The listing builds one solid part. Answer for the finished solid, in the listing's coordinates (mm). Round coordinates to 2 decimals unless told otherwise and drop trailing zeros. Write each loop counter-clockwise with the first axis right and the second up, starting at its lowest first coordinate (ties: lowest second). Pieces come first, ordered by that corner, then holes.
Item 1: Find section C-C on x = 45.65. Give the vertices of the cut face in (y, z).
Item 2: Find the intervals of material crossed by probe 1 along Y at (x, z) = (76.65, 1.2); probe 2 along X at (y, z) = (36.5, 0.2); probe 3 along X at (y, z) = (36.65, 0.9), in increasing order.
Item 3: Find section A-A on x = 61.15. Give the vertices of the cut face in (y, z).
Item 4: Find section B-B on y = 26.5. Give the vertices of the cut face in (x, z), then the cut area to 3 significant figures.
Item 5: Find section D-D on z = 2.15. Give the vertices of the cut face in (x, y).
Solid Edge part; units mm, degrees
sketch "Sketch1" plane through (0, 0, 0) normal (0, 0, 1) x (1, 0, 0)
  line L0 (0, 0) -> (82.3, 0)
  line L1 (82.3, 0) -> (82.3, 42.3)
  line L2 (82.3, 42.3) -> (40, 42.3)
  line L3 (40, 42.3) -> (0, 20)
  line L4 (0, 20) -> (0, 0)
extrude "Protrusion1" add sketch "Sketch1" along normal blind 4
hole "Hole_1" at (10, 10, 4) direction (0, 0, -1) diameter 8 end up to next
hole "Hole1" at (30, 10, 4) direction (0, 0, -1) diameter 8 end up to next
hole "Hole_3" at (61.15, 21.15, 4) direction (0, 0, -1) diameter 23 end up to next
hole "Hole_4" at (45.65, 36.65, 4) direction (0, 0, -1) diameter 3.2 end up to next
pattern_linear "Pattern2" count 2 spacing 31 along (1, 0, 0) count 2 spacing 31 along (0, -1, 0) of "Hole_4"
fillet "Round_1" radius 5 4 edges at (0, 20, 2) (82.3, 42.3, 2) (82.3, 0, 2) (40, 42.3, 2)
fillet "Round_2" radius 1.5 1 edges at (0, 0, 2)
properties material "Aluminum, 6061-T6"
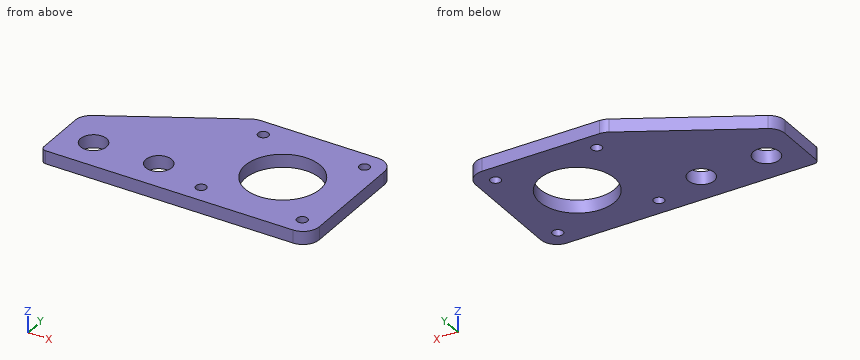
Check values:
1. outline: (0, 0) - (4.05, 0) - (4.05, 4) - (0, 4) - close; (7.25, 0) - (35.05, 0) - (35.05, 4) - (7.25, 4) - close; (38.25, 0) - (42.3, 0) - (42.3, 4) - (38.25, 4) - close
2. probe 1: y = 0 to 4.05, 7.25 to 35.05, 38.25 to 42.3
2. probe 2: x = 29.6 to 44.06, 47.24 to 75.06, 78.24 to 82.3
2. probe 3: x = 29.87 to 44.05, 47.25 to 75.05, 78.25 to 82.3
3. outline: (0, 0) - (9.65, 0) - (9.65, 4) - (0, 4) - close; (32.65, 0) - (42.3, 0) - (42.3, 4) - (32.65, 4) - close
4. outline: (11.66, 0) - (50.97, 0) - (50.97, 4) - (11.66, 4) - close; (71.33, 0) - (82.3, 0) - (82.3, 4) - (71.33, 4) - close
4. area: 201 mm2
5. outline: (0, 1.5) arc R1.5 ccw to (1.5, 0) - (77.3, 0) arc R5 ccw to (82.3, 5) - (82.3, 37.3) arc R5 ccw to (77.3, 42.3) - (41.3, 42.3) arc R5 ccw to (38.86, 41.67) - (2.57, 21.43) arc R5 ccw to (0, 17.06) - close; hole circle Ø8 at (10, 10); hole circle Ø8 at (30, 10); hole circle Ø3.2 at (45.65, 5.65); hole circle Ø3.2 at (45.65, 36.65); hole circle Ø23 at (61.15, 21.15); hole circle Ø3.2 at (76.65, 5.65); hole circle Ø3.2 at (76.65, 36.65)
